Read the model definition and answer for the solid it produces. Units are mm, in the model's axes. Face numbers are marked on the shaded views. A direction names the side the tool comes from. Coordinates: 2 decimals unless noted, no trailing zeros. Write each loop counter-clockwise with the first axis right and the second up, starting at its lowest first coordinate (ties: lowest second). Pieces come first, ordered by that corner, then holes.
(1) The part is cut by section B-B, the plane y = -21.5. Determine the outline of the cut face in (x, z).
(2) The part is cut by section D-D, the plane x = -4. Determine the outline of the cut face in (y, z).
(3) Which of the six approach directions +Z, -Z, +X, -X, +Y, -Y give full straight-line access (tool end or side, diameter ignored) to the marked faces 1, 2 and 3?
(4) The part is cut by section A-A, the plane x = -26. Determine the outline of the cut face in (y, z).
(5) The part is cut by section C-C, the plane z = 41. Determine the outline of the cut face in (x, y).
(6) Given pin 1 (3 mm diameter, centred on y = -22, z = 8.5, fed in from -X); pin 2 (2.5 mm diameter, centred on x = -28.5, y = -42, fed in from +Z); pin 3 (1.5 mm diameter, centred on y = -21.5, z = 11, fed in from +X), each flat-ended and moving along its own axis, determine where each tip first touches the part or whether it passes through.
(7) Straight lines are drawn through the part: line 1 along X through (y, z) = (-6, 25.5); line 2 along Z through (x, y) = (-21, -7). For each, find the intervals that lie inside material, in ascending order.
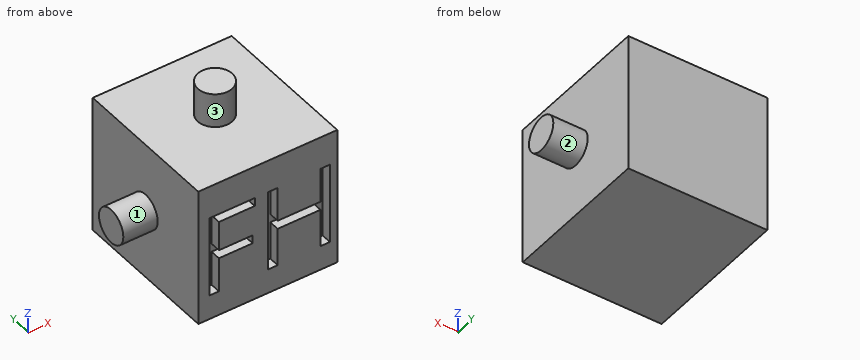
```python
from build123d import *

# Parameters (mm, degrees)
F0_W     = 40
F0_H     = 40
F1_DEPTH = 40
F2_W     = 40
F2_H     = 40
F3_DEPTH = 3
F4_R     = 4.95
F5_DEPTH = 9.9
F6_R     = 4.95
F7_DEPTH = 9.9
F8_R     = 4.95
F9_DEPTH = 9.9


with BuildPart() as f1:
    # F0 (on Front) → F1 (new body)
    with BuildSketch(Plane.XZ):
        with Locations((-20, 20)):
            Rectangle(F0_W, F0_H)
    extrude(amount=F1_DEPTH)

    # F2 (on face) → F3 (join)
    with BuildSketch(Plane.XZ.offset(40)):
        with Locations((-20, 20)):
            Rectangle(F2_W, F2_H)
        Polygon((-34.0678182981, 17.1128881329), (-34.0678182981, 7.1167269045), (-36.7856685861, 7.1167269045), (-36.7856685861, 30.5025234496), (-23.7492002559, 30.5025234496), (-23.7492002559, 28.086656527), (-34.0678182981, 28.086656527), (-34.0678182981, 19.5287550555), (-24.3736404351, 19.5287550555), (-24.3736404351, 17.1128881329), align=None, mode=Mode.SUBTRACT)
        Polygon((-2.1241202815, 30.5025234496), (-2.1241202815, 7.1167269045), (-4.8419705694, 7.1167269045), (-4.8419705694, 18.1212054714), (-17.1618682022, 18.1212054714), (-17.1618682022, 7.1167269045), (-19.8797184901, 7.1167269045), (-19.8797184901, 30.5025234496), (-17.1618682022, 30.5025234496), (-17.1618682022, 20.5524274803), (-4.8419705694, 20.5524274803), (-4.8419705694, 30.5025234496), align=None, mode=Mode.SUBTRACT)
    extrude(amount=F3_DEPTH)

    # F4 (on face) → F5 (join)
    with BuildSketch(Plane.XY.offset(40)):
        with Locations((-20, -21.5)):
            Circle(F4_R)
    extrude(amount=F5_DEPTH)

    # F6 (on face) → F7 (join)
    with BuildSketch(Plane(origin=(-40, 0, 0), x_dir=(0, -1, 0), z_dir=(-1, 0, 0))):
        with Locations((21.5, 20)):
            Circle(F6_R)
    extrude(amount=F7_DEPTH)

    # F8 (on face) → F9 (join)
    with BuildSketch(Plane.YZ):
        with Locations((-21.5, 20)):
            Circle(F8_R)
    extrude(amount=F9_DEPTH)


solid = f1.part
```
Computed:
1. outline: (-49.9, 15.05) - (-40, 15.05) - (-40, 0) - (0, 0) - (0, 15.05) - (9.9, 15.05) - (9.9, 24.95) - (0, 24.95) - (0, 40) - (-15.05, 40) - (-15.05, 49.9) - (-24.95, 49.9) - (-24.95, 40) - (-40, 40) - (-40, 24.95) - (-49.9, 24.95) - close
2. outline: (-43, 0) - (0, 0) - (0, 40) - (-43, 40) - (-43, 30.5) - (-40, 30.5) - (-40, 7.12) - (-43, 7.12) - close
3. face 1: -X
3. face 2: +X
3. face 3: +Z
4. outline: (-43, 0) - (0, 0) - (0, 40) - (-43, 40) - (-43, 30.5) - (-40, 30.5) - (-40, 28.09) - (-43, 28.09) - (-43, 19.53) - (-40, 19.53) - (-40, 17.11) - (-43, 17.11) - close
5. outline: circle Ø9.9 at (-20, -21.5)
6. pin 1: stops at x = -40
6. pin 2: stops at z = 40
6. pin 3: stops at x = 0
7. line 1: x = -40 to 0
7. line 2: z = 0 to 40
